Input: part model. Units: mm. Frame: model coordinates. Face numbers are marked on the shaded views. A direction names the side the tool comes from. Give positions to 0.01 mm unless a question says otherwise; leave off trailing zeros. Order: outer loops, then holes, each group sorted by start corner. A loop starts at its lowest first (then second) coordinate and runs counter-clockwise, first axis right, second up. Notation, with made-up numbers: M 69,83.5 L 110,83.5 A24 ccw 110,102.5 Z; hole C -32.5,24 d9. An arc over 180 degrees is marked long. Use a Markdown table: item, result.
from build123d import *

# Parameters (mm, degrees)
F1_DEPTH = 25.4
F2_R     = 5.08
F3_T     = 2.54


# Not quite as in the source:
# - a shell that OpenCascade refuses in one call is made with other operations: the cavity is built on its own and cut out


with BuildPart() as f1:
    # F0 (on Right) → F1 (new body)
    with BuildSketch(Plane.YZ):
        with BuildLine():
            ThreePointArc((-6.8017239682, 18.9395658672), (-43.2327193048, -7.2897973695), (-43.3986243496, -52.1804355085))
            Line((-43.3986243496, -52.1804355085), (59.4223327935, -52.1804355085))
            Line((59.4223327935, -52.1804355085), (59.4223327935, 0))
            ThreePointArc((59.4223327935, 0), (19.2591298188, -15.1853432617), (-6.8017239682, 18.9395658672))
        make_face()
    extrude(amount=F1_DEPTH)

    # F2
    f2_edges = [f1.edges().sort_by_distance(p)[0] for p in [
        (12.7, 59.422333, 0),
        (12.7, -6.801724, 18.939566),
        (0, 19.25913, -15.185343),
        (25.4, 19.25913, -15.185343),
    ]]
    fillet(f2_edges, radius=F2_R)

    # F3: shell of thickness 2.54, made by hand


with BuildPart() as f3_core1:
    # F3_t2: copy of F1
    add(f1.part)

    # the walls: a layer under each face that stays
    f3_faces = [f3_core1.faces().sort_by_distance(p)[0] for p in [
        (12.7, 59.4223327935, -32.5906768925),
        (0, 5.3570087404, -17.1811267303),
        (12.7, 56.5735474159, -8.4371389974),
        (12.7, 8.0118542219, -52.1804355085),
        (25.4, 5.3570087404, -17.1811267303),
        (1.4878975516, 15.4764567571, -15.4748956916),
        (12.7, -44.5374630823, -10.0289336824),
        (12.7, -8.6201931506, 17.0491329967),
        (23.9121024484, 15.4766540031, -15.4749730413),
    ]]
    thicken(f3_faces, amount=-F3_T, mode=Mode.SUBTRACT)


with BuildPart() as f1_1:
    add(f1.part)

    # what is left inside the walls is the cavity
    f3_cavity = [f3_core1.part.solids().sort_by_distance(p)[0] for p in [
        (22.8346, 5.357009, -27.999693),
    ]]
    add(f3_cavity, mode=Mode.SUBTRACT)


solid = f1_1.part
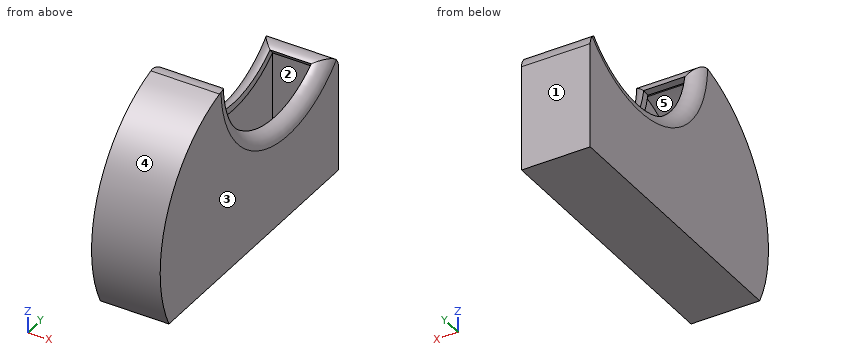
1) Material intervals for line 1 (X direction, y = 35, z = -48); line 2 (Z direction, x = 14.75, y = 39.5); line 3 (Y direction, x = 9, z = -9), sorted ascending. Write a range as from..to.
Response values:
| item | result |
|---|---|
| line 1 | x = 0..2.54, 22.86..25.4 |
| line 2 | z = -52.18..-49.64 |
| line 3 | y = -44.07..-41.25, 51.23..57.47 |
2) Cut plane B-B on z = -29.5. Return loops of the section in (x, y).
Response values:
| item | result |
|---|---|
| outline | M 0,-48.71 L 25.4,-48.71 L 25.4,59.42 L 0,59.42 Z; hole M 2.54,-46.17 L 22.86,-46.17 L 22.86,56.88 L 2.54,56.88 Z |
3) Reachability of the marked faces 4 and 5 from +Z, -Z, +X, -X, +Y, -Y: full face, straight path, thin tool, end or side. Return the list, or none.
Response values:
| item | result |
|---|---|
| face 4 | +X, -X, -Y |
| face 5 | none |
4) Mould query, pull axis X, two halves, no side actions, for the marked faces 1, 2 and 3. Classes: released by +X, released by -X, zero draft, split by the parting line, or undercut.
Response values:
| item | result |
|---|---|
| face 1 | zero draft |
| face 2 | undercut |
| face 3 | released by +X |
5) First-contact query: pin 1 Ø8 at (x, z) = (21, 1) entering from -Y; pin 2 Ø1 at (x, z) = (3.5, 2) entering from +Y; pin 3 Ø2 at (x, z) = (22.5, 6.5) entering from -Y. Flat tips, straight axial feed; report the tip coordinate or a pass-through.
Response values:
| item | result |
|---|---|
| pin 1 | stops at y = -40.75 |
| pin 2 | stops at y = -2.29 |
| pin 3 | stops at y = -33.77 |
6) Cut plane A-A on y = -28.5. Return loops of the section in (x, z).
Response values:
| item | result |
|---|---|
| outline | M 0,-52.18 L 25.4,-52.18 L 25.4,9.96 L 0,9.96 Z; hole M 2.54,-49.64 L 22.86,-49.64 L 22.86,6.76 L 2.54,6.76 Z |
